from build123d import *

# Parameters (mm, degrees)
CHAMFER1_SIZE      = 0.5
SKETCH2_W          = 3.5
SKETCH2_H          = 12
CUT_EXTRUDE1_DEPTH = 4


with BuildPart() as part:
    # Sketch1 → Revolve1 (revolve)
    with BuildSketch(Plane.XY):
        Polygon((0, -6), (0, 0), (233, 0), (233, -3), (218.5, -3), (218, -2.5), (217, -2.5), (217, -3), (19, -3), (19, -6), align=None)
    revolve(axis=Axis((-26.391164048, 0, 0), (1, 0, 0)))

    # Chamfer1
    chamfer1_edges = [part.edges().sort_by_distance(p)[0] for p in [
        (233, 3, 0),
    ]]
    chamfer(chamfer1_edges, length=CHAMFER1_SIZE)

    # Sketch2 → Cut-Extrude1 (cut)
    with BuildSketch(Plane(origin=(217, 0, 0), x_dir=(0, 0, -1), z_dir=(1, 0, 0))):
        with Locations((-4.25, 0)):
            Rectangle(SKETCH2_W, SKETCH2_H)
    cut_extrude1 = extrude(amount=-CUT_EXTRUDE1_DEPTH, mode=Mode.SUBTRACT)

    # Mirror1: Cut-Extrude1 across plane
    add(cut_extrude1.mirror(Plane.XY), mode=Mode.SUBTRACT)


solid = part.part
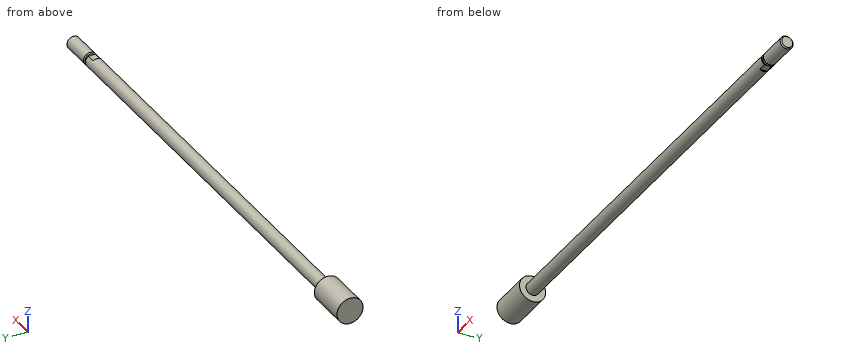
Check sheet for the modelled part. Datum: model origin and axes. Units: mm. Give positions to 0.01 mm unless a question says otherwise; leave off trailing zeros. Loops run counter-clockwise (first coordinate to the right, second up) from the corner with the lowest first, then second, coordinate; pieces in that order, holes last. Notation, with made-up numbers: M -39.5,50 L -3.5,50 A18 cw -3.5,64 Z; hole C 87.25,76.5 d2. An arc over 180 degrees is marked long. Answer as a JSON object with one key per item and string values. Group by question number.
Q1. Go/stop test with flat-tipped pins: P1, Ø2.5, axis at x = 216, y = 0, coming from the +Z side; P2, Ø6, axis at x = 206, z = -1.5, coming from the -Y side; P3, Ø1.5, axis at x = 116, y = -2, coming from the +Z side. Record where each tip stops, or that it passes through.
Q2. Material ranges on line 1 along X through (y, z) = (4.5, -3.25); line 2 along X through (y, z) = (-2.25, 1.5); line 3 along Y through (x, z) = (206, -2.5), recorded low to high. Write a range as [from, to].
Q3. Cross-section at A-A on z = 0. Record the cut outline in (x, y).
Q4. Cross-section at B-B on x = 145. Record the cut outline in (y, z).
Evaluation:
{
 "1": {"P1": "stops at z = 2.5", "P2": "stops at y = -3", "P3": "stops at z = 2.73"},
 "2": {"line 1": "x = [0, 19]", "line 2": "x = [0, 217], [218.2, 232.8]", "line 3": "y = [-1.66, 1.66]"},
 "3": {"outline": "M 0,-6 L 19,-6 L 19,-3 L 217,-3 L 217,-2.5 L 218,-2.5 L 218.5,-3 L 232.5,-3 L 233,-2.5 L 233,2.5 L 232.5,3 L 218.5,3 L 218,2.5 L 217,2.5 L 217,3 L 19,3 L 19,6 L 0,6 Z"},
 "4": {"outline": "C 0,0 d6"}
}
